```python
from build123d import *

# Parameters (mm, degrees)
SKETCH_1_W               = 12
SKETCH_1_H               = 8
EXTRUDE_1_DEPTH          = 2
SKETCH_3_W               = 5
SKETCH_3_H               = 5
EXTRUDE_2_DEPTH          = 7
SKETCH_5_R               = 1.25
CUT_EXTRUDE_2_DEPTH      = 5
CUT_EXTRUDE_2_DEPTH_BACK = 5
SKETCH_6_W               = 3.5
SKETCH_6_H               = 5
EXTRUDE_3_DEPTH          = 7
SKETCH_8_R               = 0.9
CUT_EXTRUDE_3_DEPTH      = 7
CUT_EXTRUDE_3_DEPTH_BACK = 7


with BuildPart() as part:
    # 草圖1 → 填料-伸長1 (new body)
    with BuildSketch(Plane.XY):
        with Locations((1.458189105, 0.025974026)):
            Rectangle(SKETCH_1_W, SKETCH_1_H)
    extrude(amount=EXTRUDE_1_DEPTH)

    # 草圖3 → 填料-伸長2 (add)
    with BuildSketch(Plane.XY):
        with Locations((-1.465017587, 0.025974026)):
            Rectangle(SKETCH_3_W, SKETCH_3_H)
    extrude(amount=EXTRUDE_2_DEPTH)

    # 草圖5 → 除料-伸長2 (cut, two sides)
    with BuildSketch(Plane(origin=(0, 0, 0), x_dir=(1, 0, 0), z_dir=(0, 1, 0))) as cut_extrude_2_sk:
        with Locations((-1.465017587, -4.5)):
            Circle(SKETCH_5_R)
    extrude(amount=CUT_EXTRUDE_2_DEPTH, mode=Mode.SUBTRACT)
    extrude(cut_extrude_2_sk.sketch, amount=-CUT_EXTRUDE_2_DEPTH_BACK, mode=Mode.SUBTRACT)

    # 草圖6 → 填料-伸長3 (add)
    with BuildSketch(Plane.XY):
        with Locations((5.183136142, 0.079162411)):
            Rectangle(SKETCH_6_W, SKETCH_6_H)
    extrude(amount=EXTRUDE_3_DEPTH)

    # 草圖8 → 除料-伸長3 (cut, two sides)
    with BuildSketch(Plane(origin=(0, 0, 0), x_dir=(1, 0, 0), z_dir=(0, 1, 0))) as cut_extrude_3_sk:
        with Locations((5.184982413, -4.5)):
            Circle(SKETCH_8_R)
    extrude(amount=CUT_EXTRUDE_3_DEPTH, mode=Mode.SUBTRACT)
    extrude(cut_extrude_3_sk.sketch, amount=-CUT_EXTRUDE_3_DEPTH_BACK, mode=Mode.SUBTRACT)


solid = part.part
```
Geometry check sheet. Reference: the model listing, model coordinates, mm. A direction names the side the tool comes from. Round coordinates to 2 decimals unless told otherwise and drop trailing zeros. Loops run counter-clockwise (first coordinate to the right, second up) from the corner with the lowest first, then second, coordinate; pieces in that order, holes last. Notation, with made-up numbers: (86, 0) - (125, 0) arc R14 ccw to (125, 14) - close; hole circle Ø2 at (9.25, 69). An arc over 180 degrees is marked (long way). Write item = value, one per line. Start each with the question number.
1. Mould release check, pull along X, two halves, no side actions. Record for faces 4 (the face through (7.458, 0, 1)), 5 (the face through (3.433, 0, 4)), 6 (the face through (1, 4.026, 1)): released by +X, released by -X, zero draft, split by the parting line, or undercut.
2. Set-up check for faces 1 (the face through (-3.965, 0, 4)), 2 (the face through (1.035, 0, 4)), 3 (the face through (-3, 2.526, 4)): record each of +Z, -Z, +X, -X, +Y, -Y from which the full face is reachable in a straight line by a thin tool's end or side.
3. Section check A-A on z = 2.75. Enter the section's corners in (x, y).
4. Section check C-C on y = -1.75. Enter the section's corners in (x, z).
5. Depth check by flat-ended pin: pin 1 (4 mm diameter, centred on y = 0.5, z = 4.5, fed in from -X) (3 decimals); pin 2 (1.5 mm diameter, centred on y = 0.5, z = 4.5, fed in from +X); pin 3 (1.5 mm diameter, centred on x = -1.47, z = 4.5, fed in from +Y); pin 4 (2.5 mm diameter, centred on x = -1.5, z = 4, fed in from -Y). Enter the tip coordinate at first touch or a pass-through.
6. Thickness scan on line 1 (X direction, y = -0.85, z = 4.5); line 2 (Z direction, x = 5.25, y = 1.25); line 3 (X direction, y = -1.25, z = 6). Record the ranges inside material, lowest first.
7. Section check D-D on x = 0.75. Enter the section's corners in (y, z), then the cut area to 3 significant figures.
8. Section check B-B on z = 4.5. Enter the section's corners in (x, y), then the cut area to 3 significant figures.
Working result:
q1.face_4 = released by +X
q1.face_5 = undercut
q1.face_6 = zero draft
q2.face_1 = +Z, -X, +Y, -Y
q2.face_2 = +Z, +Y, -Y
q2.face_3 = +Z, -X, +Y
q3.outline = (-3.97, -2.47) - (1.03, -2.47) - (1.03, 2.53) - (-3.97, 2.53) - close; (3.43, -2.42) - (6.93, -2.42) - (6.93, 2.58) - (3.43, 2.58) - close
q4.outline = (-4.54, 0) - (7.46, 0) - (7.46, 2) - (6.93, 2) - (6.93, 7) - (3.43, 7) - (3.43, 2) - (1.03, 2) - (1.03, 7) - (-3.97, 7) - (-3.97, 2) - (-4.54, 2) - close; hole circle Ø2.5 at (-1.47, 4.5); hole circle Ø1.8 at (5.18, 4.5)
q5.pin_1 = -3.965
q5.pin_2 = 6.93
q5.pin_3 = through
q5.pin_4 = -2.47
q6.line_1 = -3.97 to -2.72, -0.22 to 1.03, 3.43 to 4.28, 6.08 to 6.93
q6.line_2 = 0 to 3.6, 5.4 to 7
q6.line_3 = -3.97 to 1.03, 3.43 to 6.93
q7.outline = (-3.97, 0) - (4.03, 0) - (4.03, 2) - (2.53, 2) - (2.53, 7) - (-2.47, 7) - (-2.47, 2) - (-3.97, 2) - close
q7.area = 41.0 mm^2
q8.outline = (-3.97, -2.47) - (-2.72, -2.47) - (-2.72, 2.53) - (-3.97, 2.53) - close; (-0.22, -2.47) - (1.03, -2.47) - (1.03, 2.53) - (-0.22, 2.53) - close; (3.43, -2.42) - (4.28, -2.42) - (4.28, 2.58) - (3.43, 2.58) - close; (6.08, -2.42) - (6.93, -2.42) - (6.93, 2.58) - (6.08, 2.58) - close
q8.area = 21.0 mm^2
